Geometry check sheet. Reference: the model listing, model coordinates, mm. Face numbers are marked on the shaded views. A direction names the side the tool comes from. Coordinates: 2 decimals unless noted, no trailing zeros. Loops run counter-clockwise (first coordinate to the right, second up) from the corner with the lowest first, then second, coordinate; pieces in that order, holes last. Notation, with made-up numbers: M 72,29.25 L 127,29.25 A9 cw 127,42.25 Z; hole C 54.25,83.5 d6. An arc over 180 degrees is marked long. One line per question, with ' | ' between items. Start each with the question number.
from build123d import *

# Parameters (mm, degrees)
F0_R     = 30
F0_R_2   = 2.5
F1_DEPTH = 20
F2_W     = 31
F2_H     = 31
F3_DEPTH = 20.001
F4_R     = 2
F5_DEPTH = 20.001
F6_R     = 5


with BuildPart() as f1:
    # F0 (on Front) → F1 (new body)
    with BuildSketch(Plane.XZ):
        Circle(F0_R)
        with Locations((0, -25.5)):
            Circle(F0_R_2, mode=Mode.SUBTRACT)
        with Locations((-25.5, 0)):
            Circle(F0_R_2, mode=Mode.SUBTRACT)
        with Locations((25.5, 0)):
            Circle(F0_R_2, mode=Mode.SUBTRACT)
        with Locations((0, 25.5)):
            Circle(F0_R_2, mode=Mode.SUBTRACT)
    extrude(amount=F1_DEPTH)

    # F2 (on Front) → F3 (cut, through all)
    with BuildSketch(Plane.XZ):
        Rectangle(F2_W, F2_H)
    extrude(amount=F3_DEPTH, mode=Mode.SUBTRACT)

    # F4 (on Front) → F5 (cut, through all)
    with BuildSketch(Plane.XZ):
        with Locations((-14.5, 14.5)):
            Circle(F4_R)
        with Locations((14.5, 14.5)):
            Circle(F4_R)
        with Locations((14.5, -14.5)):
            Circle(F4_R)
        with Locations((-14.5, -14.5)):
            Circle(F4_R)
    extrude(amount=F5_DEPTH, mode=Mode.SUBTRACT)

    # F6
    f6_edges = [f1.edges().sort_by_distance(p)[0] for p in [
        (-12.767949, -10, 15.5),
        (-15.5, -10, 12.767949),
        (-15.5, -10, -12.767949),
        (-12.767949, -10, -15.5),
        (12.767949, -10, -15.5),
        (15.5, -10, -12.767949),
        (15.5, -10, 12.767949),
        (12.767949, -10, 15.5),
    ]]
    fillet(f6_edges, radius=F6_R)


solid = f1.part
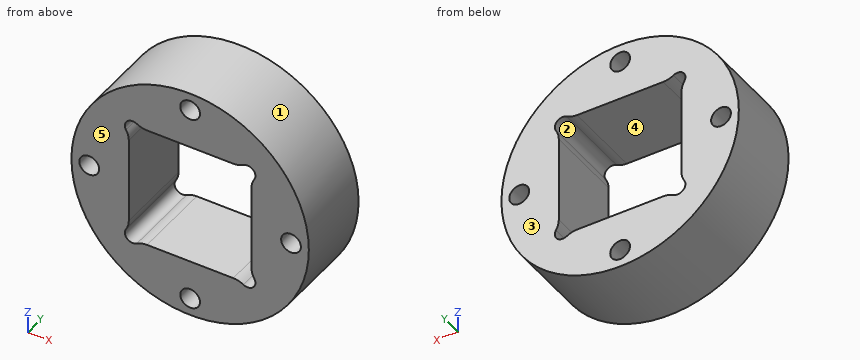
1. Sectioned sample at A-A (z = 0). Record the cut outline in (x, y).
2. Draft check along X on the marked faces 1, 2 and 3. Enter one of: +X half, -X half, draft (parallel to the pull), parting line (faces both ways), or undercut.
3. Sectioned sample at C-C (y = -18.5). Record the cut outline in (x, z), and give its area (3 significant figures).
4. Sectioned sample at D-D (x = -25.5). Record the cut outline in (y, z), and give its area (3 significant figures).
5. Thickness scan on line 1 (Z direction, x = 0, y = -5); line 2 (Z direction, x = -0.5, y = -7.5); line 3 (X direction, y = -11.5, z = -1). Record the ranges inside material, lowest first.
6. Sectioned sample at B-B (x = 0). Record the cut outline in (y, z), and give its area (3 significant figures).
7. Tool access check on the marked faces 4 and 5. Record the directions out of +Z, -Z, +X, -X, +Y, -Y that give a thin tool (end or side, any length) a straight path to the whole face; none if there is none.
8. Depth check by flat-ended pin: pin 1 Ø6 at (y, z) = (-4, 15.5) entering from +X; pin 2 Ø5 at (x, y) = (-17, -16) entering from +Z; pin 3 Ø6 at (x, y) = (0.5, -6.5) entering from +Z; pin 4 Ø3 at (x, z) = (15, 19) entering from +Y. Enter the tip coordinate at first touch or a pass-through.
Result:
1) outline: M -30,-20 L -28,-20 L -28,0 L -30,0 Z; M -23,-20 L -15.5,-20 L -15.5,0 L -23,0 Z; M 15.5,-20 L 23,-20 L 23,0 L 15.5,0 Z; M 28,-20 L 30,-20 L 30,0 L 28,0 Z
2) face 1: parting line | face 2: undercut | face 3: draft
3) outline: C 0,0 d60; hole C -25.5,0 d5; hole M -16.21,-13.47 A2 ccw -13.47,-16.21 A5 cw -10.89,-15.5 L 10.89,-15.5 A5 cw 13.47,-16.21 A2 ccw 16.21,-13.47 A5 cw 15.5,-10.89 L 15.5,10.89 A5 cw 16.21,13.47 A2 ccw 13.47,16.21 A5 cw 10.89,15.5 L -10.89,15.5 A5 cw -13.47,16.21 A2 ccw -16.21,13.47 A5 cw -15.5,10.89 L -15.5,-10.89 A5 cw Z; hole C 0,-25.5 d5; hole C 0,25.5 d5; hole C 25.5,0 d5 | area: 1,770 mm2
4) outline: M -20,-15.8 L 0,-15.8 L 0,-2.5 L -20,-2.5 Z; M -20,2.5 L 0,2.5 L 0,15.8 L -20,15.8 Z | area: 532 mm2
5) line 1: z = -30 to -28, -23 to -15.5, 15.5 to 23, 28 to 30 | line 2: z = -30 to -27.95, -23.05 to -15.5, 15.5 to 23.05, 27.95 to 30 | line 3: x = -29.98 to -27.79, -23.21 to -15.5, 15.5 to 23.21, 27.79 to 29.98
6) outline: M -20,-30 L 0,-30 L 0,-28 L -20,-28 Z; M -20,-23 L 0,-23 L 0,-15.5 L -20,-15.5 Z; M -20,15.5 L 0,15.5 L 0,23 L -20,23 Z; M -20,28 L 0,28 L 0,30 L -20,30 Z | area: 380 mm2
7) face 4: +Y, -Y | face 5: +Z, -Z, +X, -X, -Y
8) pin 1: stops at x = 27.27 | pin 2: stops at z = 26.26 | pin 3: stops at z = 30 | pin 4: stops at y = 0
